Part model, mm, in its own coordinate system. Round coordinates to 2 decimals unless told otherwise and drop trailing zeros. Loops run counter-clockwise (first coordinate to the right, second up) from the corner with the lowest first, then second, coordinate; pieces in that order, holes last.
1) Band-saw the part on C-C, the plane x = 2. Write the cut outline in (y, z), then the cut area to 3 significant figures.
2) Drop flat-ended pins along their axis: P1, Ø0.8, axis at y = 1, z = -34.5, coming from the -X side; P2, Ø1.1, axis at x = 0.5, y = 1, coming from the -Z side; P3, Ø0.5, axis at x = 17, y = 1, coming from the -Z side. Give the stop position or say it passes through.
3) Probe line 1 (Z direction, x = 11.75, y = 0.9); line 2 (Z direction, x = 15.75, y = 0.9); line 3 (X direction, y = 0.95, z = 0.5). List the from-to ranges inside material, lowest first.
4) Band-saw the part on B-B, the plane y = 1.1. Write the cut outline in (x, z).
5) Band-saw the part on A-A, the plane x = 7.25. Write the cut outline in (y, z), then the cut area to 3 significant figures.
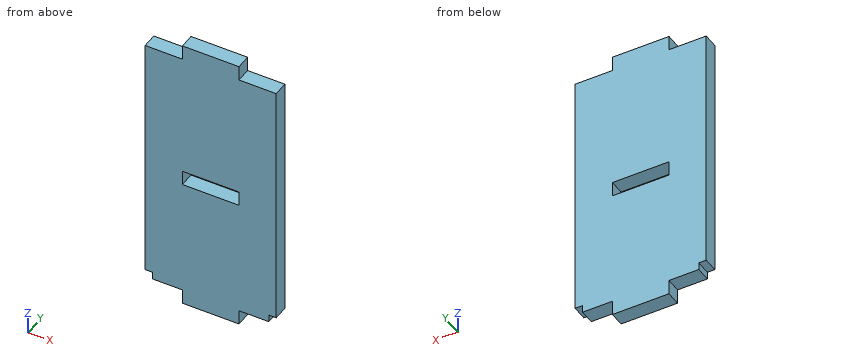
from build123d import *

# Parameters (mm, degrees)
SKETCH_1_W      = 7.6
SKETCH_1_H      = 2
EXTRUDE_1_DEPTH = 2


with BuildPart() as part:
    # 草图1 → 凸台-拉伸1 (new body)
    with BuildSketch(Plane(origin=(0, 0, 0), x_dir=(1, 0, 0), z_dir=(0, 1, 0))):
        Polygon((0, 33.8), (0, 0), (5, 0), (5, -2), (12.6, -2), (12.6, 0), (17.6, 0), (17.6, 33.8), (16.6, 33.8), (16.6, 34.8), (12.6, 34.8), (12.6, 36.8), (5, 36.8), (5, 34.8), (1, 34.8), (1, 33.8), align=None)
        with Locations((8.8, 17.9)):
            Rectangle(SKETCH_1_W, SKETCH_1_H, mode=Mode.SUBTRACT)
    extrude(amount=EXTRUDE_1_DEPTH)


solid = part.part
Reported:
1. outline: (0, -34.8) - (2, -34.8) - (2, 0) - (0, 0) - close
1. area: 69.6 mm2
2. P1: stops at x = 1
2. P2: stops at z = -34.8
2. P3: stops at z = -33.8
3. line 1: z = -36.8 to -18.9, -16.9 to 2
3. line 2: z = -34.8 to 0
3. line 3: x = 5 to 12.6
4. outline: (0, -33.8) - (1, -33.8) - (1, -34.8) - (5, -34.8) - (5, -36.8) - (12.6, -36.8) - (12.6, -34.8) - (16.6, -34.8) - (16.6, -33.8) - (17.6, -33.8) - (17.6, 0) - (12.6, 0) - (12.6, 2) - (5, 2) - (5, 0) - (0, 0) - close; hole (5, -18.9) - (12.6, -18.9) - (12.6, -16.9) - (5, -16.9) - close
5. outline: (0, -36.8) - (2, -36.8) - (2, -18.9) - (0, -18.9) - close; (0, -16.9) - (2, -16.9) - (2, 2) - (0, 2) - close
5. area: 73.6 mm2
